Check sheet for the drawn part. Datum: minimum x, y, z corner. Units: mm. A direction names the side the tool comes from. Give positions to 0.01 mm unless a question says otherwise; leave off trailing zeros. Write each loop counter-clockwise with the first axis right and the second up, starting at its lowest first coordinate (ties: lowest second). Pieces come first, ordered by that corner, then holes. Notation, with made-up numbers: (-3, 74.25) - (16, 74.25) arc R35 cw to (16, 106.25) - close; hole circle Ø6 at (48, -19.5). An arc over 180 degrees is marked (long way). Use a Markdown table: item, result.
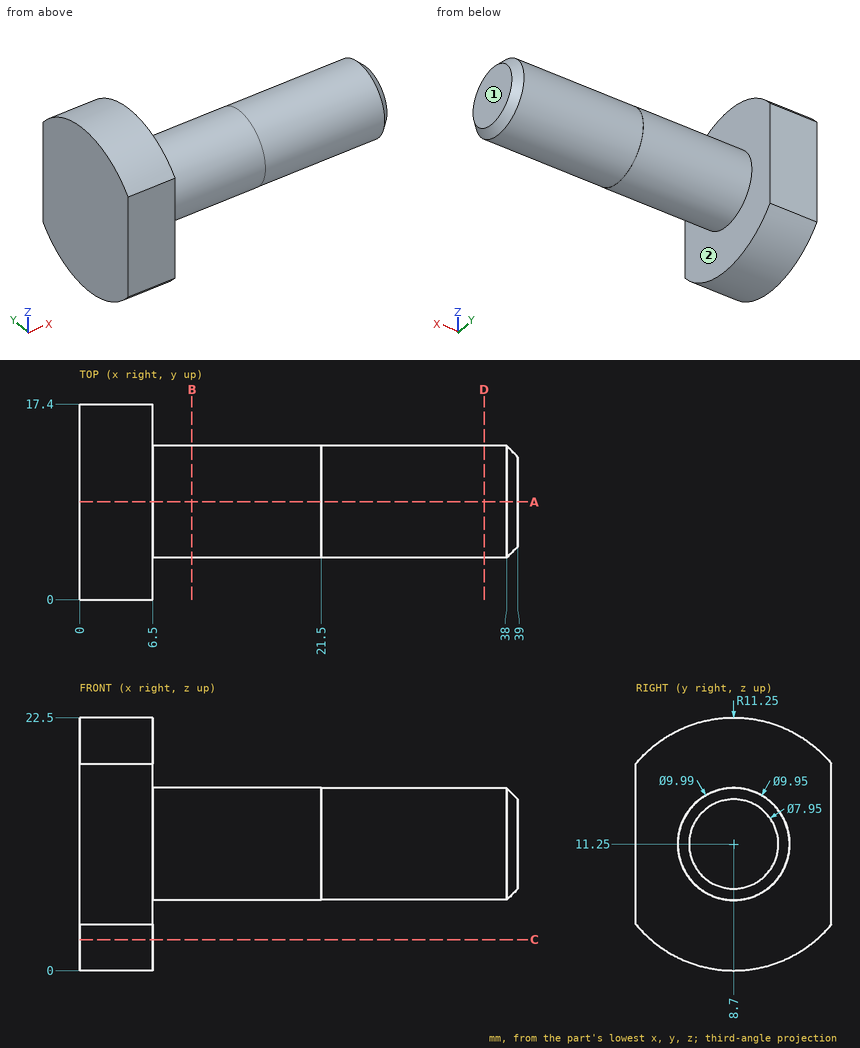
1) Section check C-C on z = 2.75. Record the boundary of the cut face in (x, y), then the cut area to 3 significant figures.
Working result:
| item | result |
|---|---|
| outline | (0, 1.33) - (6.5, 1.33) - (6.5, 16.07) - (0, 16.07) - close |
| area | 95.8 mm² |
2) Depth check by flat-ended pin: P1, Ø1, axis at y = 5.5, z = 5, coming from the +X side; P2, Ø2, axis at x = 14.5, y = 10, coming from the -Z side; P3, Ø10, axis at x = 24.5, y = 11.5, coming from the +Z side (3 decimals); P4, Ø3, axis at x = 6, y = 7.5, coming from the +Z side. Enter the tip coordinate at first touch or a pass-through.
Working result:
| item | result |
|---|---|
| P1 | stops at x = 6.5 |
| P2 | stops at z = 6.26 |
| P3 | stops at z = 16.245 |
| P4 | stops at z = 22.5 |
3) Section check D-D on x = 36. Record the boundary of the cut face in (y, z) (3 decimals), then the cut area to 3 significant figures.
Working result:
| item | result |
|---|---|
| outline | circle Ø9.95 at (8.7, 11.25) |
| area | 77.8 mm² |
4) Material ranges on L1, parallel to X at y = 2.5, z = 12.5; L2, parallel to Z at x = 21, y = 8.5; L3, parallel to Z at x = 2, y = 4.5, recorded low to high. Write a range as from..to.
Working result:
| item | result |
|---|---|
| L1 | x = 0..6.5 |
| L2 | z = 6.26..16.24 |
| L3 | z = 0.81..21.69 |
5) Set-up check for the marked faces 1 and 2: record each of +Z, -Z, +X, -X, +Y, -Y from which the full face is reachable in a straight line by a thin tool's end or side.
Working result:
| item | result |
|---|---|
| face 1 | +Z, -Z, +X, +Y, -Y |
| face 2 | +X |
6) Section check A-A on y = 8.7. Record the boundary of the cut face in (x, z) (3 decimals), then the cut area to 3 significant figures.
Working result:
| item | result |
|---|---|
| outline | (0, 0) - (6.5, 0) - (6.5, 6.255) - (21.5, 6.255) - (21.5, 6.275) - (38, 6.275) - (39, 7.275) - (39, 15.225) - (38, 16.225) - (21.5, 16.225) - (21.5, 16.245) - (6.5, 16.245) - (6.5, 22.5) - (0, 22.5) - close |
| area | 469 mm² |
7) Section check B-B on x = 10. Record the boundary of the cut face in (y, z) (3 decimals), then the cut area to 3 significant figures.
Working result:
| item | result |
|---|---|
| outline | circle Ø9.99 at (8.7, 11.25) |
| area | 78.4 mm² |
